Work out the finished part from the listing and answer in its coordinate system (mm). Face numbers are marked on the shaded views. A direction names the side the tool comes from. Coordinates: 2 decimals unless noted, no trailing zeros. Order: outer loops, then holes, each group sorted by start corner. A loop starts at its lowest first (then second) coordinate and runs counter-clockwise, first axis right, second up.
```python
from build123d import *

# Parameters (mm, degrees)
F1_DEPTH = 152.4
F2_DEPTH = 107.95
F0_R     = 44.45
F3_DEPTH = 127
F4_DEPTH = 19.05


with BuildPart() as f1:
    # F0 (on Front) → F1 (new body)
    with BuildSketch(Plane.XZ):
        Polygon((127, -203.2), (127, -152.4), (9.525, -152.4), (-9.525, -152.4), (-127, -152.4), (-127, -203.2), align=None)
    extrude(amount=F1_DEPTH)

    # F0 (on Front) → F2 (join)
    with BuildSketch(Plane.XZ):
        with BuildLine():
            Line((9.525, -152.4), (9.525, -62.781561))
            ThreePointArc((9.525, -62.781561), (0, -63.5), (-9.525, -62.781561))
            Line((-9.525, -62.781561), (-9.525, -152.4))
            Line((-9.525, -152.4), (9.525, -152.4))
        make_face()
    extrude(amount=F2_DEPTH)

    # F0 (on Front) → F3 (join)
    with BuildSketch(Plane.XZ):
        with BuildLine():
            ThreePointArc((9.525, -62.781561), (48.151259, -41.396935), (63.5, 0))
            ThreePointArc((63.5, 0), (0, 63.5), (-63.5, 0))
            ThreePointArc((-63.5, 0), (-48.151259, -41.396935), (-9.525, -62.781561))
            ThreePointArc((-9.525, -62.781561), (0, -63.5), (9.525, -62.781561))
        make_face()
        Circle(F0_R, mode=Mode.SUBTRACT)
    extrude(amount=F3_DEPTH)

    # F0 (on Front) → F4 (join)
    with BuildSketch(Plane.XZ):
        with BuildLine():
            ThreePointArc((-9.525, -62.781561), (-48.151259, -41.396935), (-63.5, 0))
            Line((-63.5, 0), (-127, -152.4))
            Line((-127, -152.4), (-9.525, -152.4))
            Line((-9.525, -152.4), (-9.525, -62.781561))
        make_face()
        with BuildLine():
            Line((127, -152.4), (63.5, 0))
            ThreePointArc((63.5, 0), (48.151259, -41.396935), (9.525, -62.781561))
            Line((9.525, -62.781561), (9.525, -152.4))
            Line((9.525, -152.4), (127, -152.4))
        make_face()
    extrude(amount=F4_DEPTH)


solid = f1.part
```
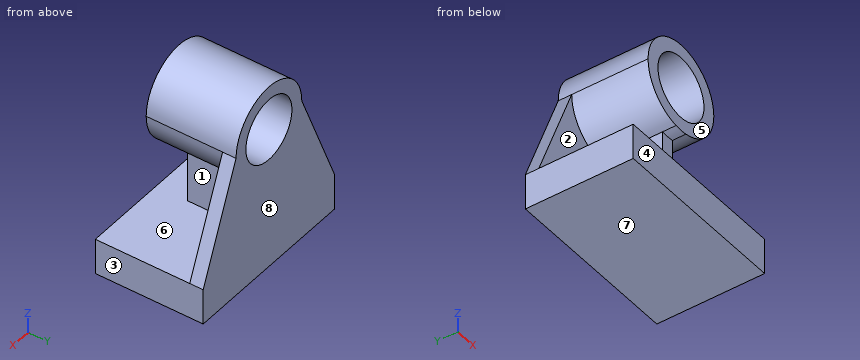
1. Consider probe 1 along Z at (x, y) = (0, -44.5); probe 2 along Z at (x, y) = (-34, -96.5); probe 3 along Z at (x, y) = (-21, -66). Determine where each line is inside the solid, lowest interval first.
2. The mould has two halves that part along Z. Classify the marked faces 6, 7 and 8: released by +Z, released by -Z, zero draft, split by the parting line, or undercut.
3. For the marked faces 1, 2, 3, 4 and 5, determine the directions among +Z, -Z, +X, -X, +Y, -Y from which every point of the face is accessible in a straight line to the end or side of a thin tool.
4. The part is cut by section A-A (y = -112). Determine the outline of the cut face in (x, z) (3 decimals), plus the area to 3 significant figures.
5. The part is cut by section C-C (y = -76). Determine the outline of the cut face in (x, z) (3 decimals), plus the area to 3 significant figures.
6. The part is cut by section D-D (z = 8.5). Determine the outline of the cut face in (x, y).
7. The part is cut by section B-B (x = 0). Determine the outline of the cut face in (y, z), plus the area to 3 significant figures.
8. Flat-ended cylindrical pins translate along their axes: pin 1 (1 mm diameter, centred on x = 57, y = -84.5, fed in from +Z); pin 2 (10 mm diameter, centred on y = -43.5, z = -122, fed in from +X) (3 decimals); pin 3 (5.5 mm diameter, centred on x = 2, z = -106, fed in from -Y). Find the tip coordinate at first contact, or state that the pin passes through.
Worked out:
1. probe 1: z = -203.2 to -44.45, 44.45 to 63.5
1. probe 2: z = -203.2 to -152.4, -53.63 to -28.63, 28.63 to 53.63
1. probe 3: z = -203.2 to -152.4, -59.93 to -39.18, 39.18 to 59.93
2. face 6: undercut
2. face 7: released by -Z
2. face 8: zero draft
3. face 1: +X, -Y
3. face 2: -X, -Y
3. face 3: +Z, -Z, +X, +Y, -Y
3. face 4: +Z, -Z, +X, -X, -Y
3. face 5: +Z, +X, -X, -Y
4. outline: (-127, -203.2) - (127, -203.2) - (127, -152.4) - (-127, -152.4) - close; (-63.5, 0) arc R63.5 ccw to (-9.525, -62.782) arc R63.5 ccw to (9.525, -62.782) arc R63.5 ccw to (63.5, 0) arc R63.5 ccw to start; hole circle Ø88.9 at (0, 0)
4. area: 19,400 mm2
5. outline: (-127, -203.2) - (127, -203.2) - (127, -152.4) - (9.525, -152.4) - (9.525, -62.782) arc R63.5 ccw to (63.5, 0) arc R63.5 ccw to (-63.5, 0) arc R63.5 ccw to (-9.525, -62.782) - (-9.525, -152.4) - (-127, -152.4) - close; hole circle Ø88.9 at (0, 0)
5. area: 21,100 mm2
6. outline: (-62.93, -127) - (-43.63, -127) - (-43.63, 0) - (-62.93, 0) - close; (43.63, -127) - (62.93, -127) - (62.93, 0) - (43.63, 0) - close
7. outline: (-152.4, -203.2) - (0, -203.2) - (0, -44.45) - (-127, -44.45) - (-127, -63.5) - (-107.95, -63.5) - (-107.95, -152.4) - (-152.4, -152.4) - close; (-127, 44.45) - (0, 44.45) - (0, 63.5) - (-127, 63.5) - close
7. area: 22,200 mm2
8. pin 1: stops at z = 28.98
8. pin 2: stops at x = 9.525
8. pin 3: stops at y = -107.95
